For this review, take the finished solid that the model builds, in its own axes (mm). A direction names the side the tool comes from. Coordinates: 2 decimals unless noted, no trailing zeros. Order: outer loops, then holes, each group sorted by start corner. A loop starts at its lowest first (then second) coordinate and runs counter-clockwise, first axis right, second up. Notation, with made-up numbers: (66.25, 14.5) - (107.25, 14.5) arc R23 cw to (107.25, 35.5) - close; hole circle Ø11 at (73.5, 51). An arc over 180 degrees is marked (long way). One line per item, written item: value. Start each with the question number.
(1) Consider section A-A on z = 10. Write out the cut boundary in (x, y).
(2) Clearance check with flat-ended pins moving along their axes: pin 1 (6 mm diameter, centred on x = -16, y = 6, fed in from +Z); pin 2 (2 mm diameter, centred on x = 13, y = -22.5, fed in from +Z); pin 3 (2 mm diameter, centred on y = 5.5, z = 10, fed in from +X); pin 4 (6 mm diameter, centred on x = 11.5, z = 9.5, fed in from -Y). State where each tip first meets the part, or that it passes through.
(3) Mouldability with a two-part tool opening along X and no side actions: class faces 4 (the flat face through (-11.69, -8.86, 1.01)), 5 (the flat face through (-15.6, 24.4, 13)), 6 (the flat face through (-8.62, 11.45, 1.01)), 7 (the cylindrical face through (-6.894, 31.044, 6.437)) as released by +X, released by -X, zero draft, split by the parting line, or undercut.
(4) To check wall thickness, follow line 1 along Y through (x, z) = (0, 9.5); line 2 along X through (y, z) = (1, 3.75); line 3 along X through (y, z) = (-16.5, 10.5). State the ranges of each line that lie inside material, in increasing order.
(5) Consider section B-B on x = -9.5. Count the separate pieces of the cut face and the enclosed holes in it, then the cut area to 3 significant figures.
(6) For faces 1 (the cylindrical face through (27.47, -8.65, 7.42)), 2 (the flat face through (-2, 2, 0)), 3 (the flat face through (-11.45, 8.62, 1.01)), list the 3-axis set-ups (+Z, -Z, +X, -X, +Y, -Y) from which the entire face can be reached by the end or side of a thin tool; tool diameter is ignored.
Solid Edge part; units mm, degrees
sketch "Sketch1" plane through (0, 0, 0) normal (0, 0, 1) x (1, 0, 0)
  circle A0 centre (0, 0) radius 31.8
extrude "Protrusion1" add sketch "Sketch1" along normal blind 2
sketch "Sketch2" plane through (0, 0, 0) normal (0, 0, 1) x (1, 0, 0)
  circle A0 centre (0, 0) radius 28.8
  circle A1 centre (0, 0) radius 31.8
extrude "ExtrudedProtrusion_3" add sketch "Sketch2" along normal blind 13
fillet "Round_2" radius 2 1 edges at (-31.8, 0, 0)
sketch "Sketch3" plane through (0, 0, 2) normal (0, 0, 1) x (0, 1, 0)
  circle A0 centre (0, 0) radius 2.5
extrude "ExtrudedProtrusion_4" add sketch "Sketch3" along normal blind 1.5
fillet "Round_3" radius 2 1 edges at (0, -2.5, 3.5)
fillet "Round_4" radius 2 1 edges at (-31.8, 0, 13)
sketch "Sketch4" plane through (0, 0, 2) normal (0, 0, 1) x (1, 0, 0)
  line L0 (-20.3118, -17.4834) -> (-2.8284, 0)
  line L1 (-2.8284, 0) -> (-20.3118, 17.4834)
  arc A0 (-20.3118, 17.4834) -> (-20.3118, -17.4834) centre (0, 0) ccw
  line L2 (0, -2.8284) -> (-17.4834, -20.3118)
  arc A1 (-17.4834, -20.3118) -> (17.4834, -20.3118) centre (0, 0) ccw
  line L3 (17.4834, -20.3118) -> (0, -2.8284)
  line L4 (17.4834, 20.3118) -> (0, 2.8284)
  line L5 (0, 2.8284) -> (-17.4834, 20.3118)
  arc A2 (-17.4834, 20.3118) -> (17.4834, 20.3118) centre (0, 0) cw
  line L6 (2.8284, 0) -> (20.3118, 17.4834)
  arc A3 (20.3118, 17.4834) -> (20.3118, -17.4834) centre (0, 0) cw
  line L7 (20.3118, -17.4834) -> (2.8284, 0)
extrude "ExtrudedCutout_1" cut sketch "Sketch4" against normal blind 22.2905
Geometry check:
1. outline: circle Ø63.6 at (0, 0); hole circle Ø57.6 at (0, 0)
2. pin 1: passes through
2. pin 2: stops at z = 2
2. pin 3: stops at x = 31.48
2. pin 4: stops at y = -30.64
3. face 4: undercut
3. face 5: zero draft
3. face 6: undercut
3. face 7: split by the parting line
4. line 1: y = -31.8 to -28.8, 28.8 to 31.8
4. line 2: x = -31.78 to -28.78, 28.78 to 31.78
4. line 3: x = -27.18 to -23.6, 23.6 to 27.18
5. separate pieces: 4
5. enclosed holes: 0
5. area: 110 mm^2
6. face 1: +Z
6. face 2: -Z, +X, -X, +Y, -Y
6. face 3: +Z, -Z
